Verification items for the finished model (mm, model axes). A direction names the side the tool comes from. Give positions to 0.01 mm unless a question says otherwise; leave off trailing zeros. Loops run counter-clockwise (first coordinate to the right, second up) from the corner with the lowest first, then second, coordinate; pieces in that order, holes last. Notation, with made-up numbers: (37, 65.25) -> (42, 65.25) arc R26 ccw to (42, 88.25) -> close; hole circle Ø2 at (63, -28.75). An arc over 180 degrees is marked (long way). Use one line per item in the form item = value. Start each with the question number.
from build123d import *

# Parameters (mm, degrees)
SKETCH2_W          = 15.49
SKETCH2_H          = 15.49
CUT_EXTRUDE1_DEPTH = 12.7


with BuildPart() as part:
    # Sketch1 → Revolve1 (revolve)
    with BuildSketch(Plane(origin=(0, 0, 0), x_dir=(1, 0, 0), z_dir=(0, 1, 0))):
        Polygon((0, 0), (165.1, 0), (165.1, 15.88), (12.7, 19.05), (0, 19.05), align=None)
    revolve(axis=Axis((0, 0, 0), (1, 0, 0)))

    # Sketch2 → Cut-Extrude1 (cut)
    with BuildSketch(Plane(origin=(165.1, 0, 0), x_dir=(0, 0, -1), z_dir=(1, 0, 0))):
        Rectangle(SKETCH2_W, SKETCH2_H)
    extrude(amount=-CUT_EXTRUDE1_DEPTH, mode=Mode.SUBTRACT)


solid = part.part
Item 1: Sectioned sample at A-A, the plane z = 0. Enter the section's corners in (x, y) (3 decimals).
Item 2: Draft check along Y on faces 1 (the flat face through (159, 0, 7.745)), 2 (the cylindrical face through (6.26, -11.59, 15.12)), 3 (the flat face through (0, 0, 0)). Enter one of: +Y half, -Y half, draft (parallel to the pull), parting line (faces both ways), or undercut.
Item 3: Sectioned sample at D-D, the plane x = 72. Enter the section's corners in (y, z), and give its area (3 significant figures).
Item 4: Gauge pin test, flat ends, axial feed: pin 1 Ø1 at (x, y) = (99.5, 3.5) entering from -Z; pin 2 Ø6.5 at (x, z) = (161.5, -1.5) entering from -Y; pin 3 Ø10 at (x, z) = (109, -1.5) entering from -Y; pin 4 Ø2 at (y, z) = (-10.5, 12.5) entering from +X. Record the tip position at first contact, or that the pin passes through.
Item 5: Material ranges on line 1 (X direction, y = -0.5, z = -1.5); line 2 (Y direction, x = 91.5, z = -2.5); line 3 (Z direction, x = 19, y = 4.5), recorded low to high.
Item 6: Sectioned sample at C-C, the plane x = 154. Enter the section's corners in (y, z) (3 decimals), and give its area (3 significant figures).
Item 7: Tool access check on faces 4 (the flat face through (165.1, -10, 0)), 5 (the conical face through (87.83, 5.25, -16.68)). Record the directions out of +Z, -Z, +X, -X, +Y, -Y that give a thin tool (end or side, any length) a straight path to the whole face; none if there is none.
Outcome:
q1.outline = (0, -19.05) -> (12.7, -19.05) -> (165.1, -15.88) -> (165.1, -7.745) -> (152.4, -7.745) -> (152.4, 7.745) -> (165.1, 7.745) -> (165.1, 15.88) -> (12.7, 19.05) -> (0, 19.05) -> close
q2.face_1 = undercut
q2.face_2 = parting line
q2.face_3 = draft
q3.outline = circle Ø35.63 at (0, 0)
q3.area = 997 mm^2
q4.pin_1 = -16.98
q4.pin_2 = -16.02
q4.pin_3 = -17.15
q4.pin_4 = 165.1
q5.line_1 = 0 to 152.4
q5.line_2 = -17.23 to 17.23
q5.line_3 = -18.38 to 18.38
q6.outline = circle Ø32.222 at (0, 0); hole (-7.745, -7.745) -> (7.745, -7.745) -> (7.745, 7.745) -> (-7.745, 7.745) -> close
q6.area = 575 mm^2
q7.face_4 = +Z, -Z, +X, +Y, -Y
q7.face_5 = +X
